from build123d import *

# Parameters (mm, degrees)
F0_W           = 30
F0_H           = 50
F1_DEPTH       = 30
F2_W           = 50
F2_H           = 15
F3_DEPTH       = 25
F5_W           = 55
F5_H           = 18
F6_DEPTH       = 5
F4_R           = 3
F7_DEPTH       = 50.001
F8_SIZE        = 0.5
F9_W           = 30
F9_H           = 12
F10_DEPTH      = 30.001
F11_R          = 12
F12_DEPTH      = 12.001
F12_DEPTH_BACK = 16
F13_SIZE       = 0.5
F14_R          = 8
F15_DEPTH      = 7.001


with BuildPart() as f1:
    # F0 (on Top) → F1 (new body)
    with BuildSketch(Plane.XY):
        with Locations((-15, 25)):
            Rectangle(F0_W, F0_H)
    extrude(amount=F1_DEPTH)

    # F2 (on face) → F3 (join)
    with BuildSketch(Plane.YZ):
        with Locations((25, 7.5)):
            Rectangle(F2_W, F2_H)
    extrude(amount=F3_DEPTH)

    # F5 (on face) → F6 (join)
    with BuildSketch(Plane(origin=(0, 0, 0), x_dir=(1, 0, 0), z_dir=(0, 0, -1))):
        with Locations((-2.5, -25)):
            Rectangle(F5_W, F5_H)
    extrude(amount=F6_DEPTH)

    # F4 (on face) → F7 (cut, through all)
    with BuildSketch(Plane.XZ):
        with Locations((-7.5, 24.5)):
            Circle(F4_R)
    extrude(amount=-F7_DEPTH, mode=Mode.SUBTRACT)

    # F8
    f8_edges = [f1.edges().sort_by_distance(p)[0] for p in [
        (-10.5, 0, 24.5),
        (-10.5, 50, 24.5),
    ]]
    chamfer(f8_edges, length=F8_SIZE)

    # F9 (on face) → F10 (cut, through all)
    with BuildSketch(Plane.YZ):
        with Locations((25, 24)):
            Rectangle(F9_W, F9_H)
    extrude(amount=-F10_DEPTH, mode=Mode.SUBTRACT)

    # F11 (on face) → F12 (cut, two sides)
    with BuildSketch(Plane.XY.offset(18)) as f12_sk:
        with Locations((-15, 25)):
            Circle(F11_R)
    extrude(amount=F12_DEPTH, mode=Mode.SUBTRACT)
    extrude(f12_sk.sketch, amount=-F12_DEPTH_BACK, mode=Mode.SUBTRACT)

    # F13
    f13_edges = [f1.edges().sort_by_distance(p)[0] for p in [
        (-30, 5, 30),
        (-15, 10, 30),
        (0, 5, 30),
        (-15, 0, 30),
        (-15, 40, 30),
        (-30, 45, 30),
        (-15, 50, 30),
        (0, 45, 30),
    ]]
    chamfer(f13_edges, length=F13_SIZE)

    # F14 (on face) → F15 (cut, through all)
    with BuildSketch(Plane.XY.offset(2)):
        with Locations((-15, 25)):
            Circle(F14_R)
    extrude(amount=-F15_DEPTH, mode=Mode.SUBTRACT)


solid = f1.part
Can you work these out from the model? Positions are in its coordinate system, mm. A direction names the side the tool comes from. Coordinates: 2 decimals unless noted, no trailing zeros. Write each loop counter-clockwise with the first axis right and the second up, starting at its lowest first coordinate (ties: lowest second). Pieces come first, ordered by that corner, then holes. Notation, with made-up numbers: M 69,3.25 L 119,3.25 A24 ccw 119,33.25 Z; hole C -34.75,75 d5. An arc over 180 degrees is marked long. Use one line per item in the form item = value.
Q1. If we section it at C-C (x = -15): Write out the boundary of the cut face in (y, z), then the cut area to 4 significant figures.
Model answer:
outline = M 0,0 L 16,0 L 16,-5 L 17,-5 L 17,2 L 13,2 L 13,18 L 10,18 L 10,29.5 L 9.5,30 L 0.5,30 L 0,29.5 Z; M 33,-5 L 34,-5 L 34,0 L 50,0 L 50,29.5 L 49.5,30 L 40.5,30 L 40,29.5 L 40,18 L 37,18 L 37,2 L 33,2 Z
area = 733.5 mm^2
Q2. For P1, Ø5, axis at x = 9, y = 39.5, coming from the -Z side; P2, Ø12, axis at x = -12, y = 27.5, coming from the +Z side; P3, Ø2.5, axis at x = -4.5, z = -1.5, coming from the +Y side; P4, Ø2, axis at x = 4, z = 16.5, coming from the -Y side, each with a flat end and sliding along its axis, tell me the tip position at first contact or that it passes through.
Model answer:
P1 = 0
P2 = 2
P3 = 34
P4 = through
Q3. For faces 1 (the flat face through (-3, 8, 0)), 2 (the flat face through (-15, 40, 24)), 3 (the cylindrical face through (-20.9, 30.4, -1.5)), 4 (the flat face through (-3, 42, 0)), 5 (the cylindrical face through (-17.601, 13.285, 10.112)), which set-ups out of +Z, -Z, +X, -X, +Y, -Y let a thin tool reach every point of the face, with its end or its side?
Model answer:
face_1 = -Z, +X, -X, -Y
face_2 = +Z, +X, -X
face_3 = +Z, -Z
face_4 = -Z, +X, -X, +Y
face_5 = +Z
Q4. If we section it at B-B (z = 19.5): Write out the boundary of the cut face in (x, y), then the cut area to 3 significant figures.
Model answer:
outline = M -30,0 L 0,0 L 0,10 L -30,10 Z; M -30,40 L 0,40 L 0,50 L -30,50 Z
area = 600 mm^2
Q5. I need wall thicknesses on line 1 along Y through (x, z) = (-1, 28.5); line 2 along Z through (x, y) = (-7.5, 2.5); line 3 along Z through (x, y) = (18.5, 17). Which ranges of each line are inside material? Lowest first, please. Write a range as from..to.
Model answer:
line_1 = 0..10, 40..50
line_2 = 0..21.5, 27.5..30
line_3 = -5..15
Q6. If we section it at D-D (y = 25): Write out the boundary of the cut face in (x, z).
Model answer:
outline = M -30,-5 L -23,-5 L -23,2 L -27,2 L -27,18 L -30,18 Z; M -7,-5 L 25,-5 L 25,15 L 0,15 L 0,18 L -3,18 L -3,2 L -7,2 Z
Q7. We'd pull the mould along X, two halves only. Please class faces 6 (the flat face through (0, 25, 17)), 7 (the cylindrical face through (-4.73, 5.18, 23.35)), 8 (the flat face through (-15, 10, 24)): +X half, -X half, draft (parallel to the pull), parting line (faces both ways), or undercut.
Model answer:
face_6 = +X half
face_7 = undercut
face_8 = draft
Q8. If we section it at A-A (y = 46): Write out the boundary of the cut face in (x, z).
Model answer:
outline = M -30,0 L 25,0 L 25,15 L 0,15 L 0,29.5 L -0.5,30 L -29.5,30 L -30,29.5 Z; hole C -7.5,24.5 d6
